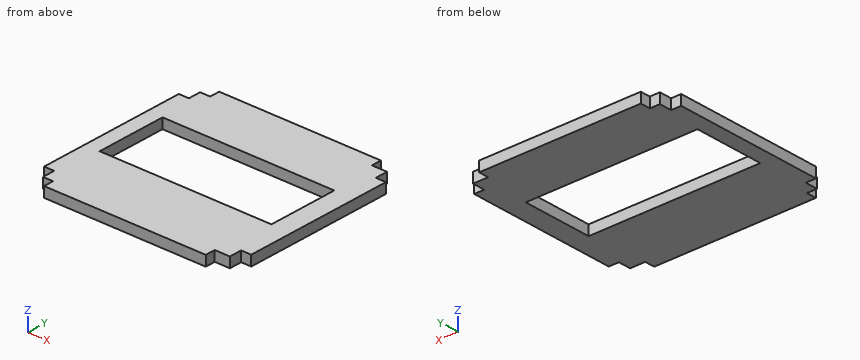
```python
from build123d import *

# Parameters (mm, degrees)
EXTRUDE_1_DEPTH = 2


with BuildPart() as part:
    # 草图1 → 凸台-拉伸1 (new body)
    with BuildSketch(Plane.XY):
        Polygon((0, -35), (2, -35), (2, -37), (34, -37), (34, -35), (37, -35), (37, -32.5), (39, -32.5), (39, -2.5), (37, -2.5), (37, 0), (34, 0), (34, 2), (2, 2), (2, 0), (0, 0), (0, -2.5), (-2, -2.5), (-2, -32.5), (0, -32.5), align=None)
        Polygon((18, -23.5), (2.5, -23.5), (1, -23.5), (1, -11.5), (1, -9.5), (35, -9.5), (35, -11.5), (35, -23.5), (33.5, -23.5), align=None, mode=Mode.SUBTRACT)
    extrude(amount=EXTRUDE_1_DEPTH)


solid = part.part
```
The listing builds one solid part. Answer for the finished solid, in the listing's coordinates (mm). Round coordinates to 2 decimals unless told otherwise and drop trailing zeros. Loops run counter-clockwise (first coordinate to the right, second up) from the corner with the lowest first, then second, coordinate; pieces in that order, holes last.
Q1. Section C-C, the plane y = -15 is taken. Determine the outline of the cut face in (x, z).
Q2. Section A-A, the plane z = 1.4 is taken. Determine the outline of the cut face in (x, y), then the cut area to 3 significant figures.
Q3. Find the intervals of material crossed by line 1 (Y direction, x = 12.5, z = 0.35); line 2 (X direction, y = -23, z = 1.65); line 3 (X direction, y = -0.5, z = 0.5), in increasing order.
Q4. Section B-B, the plane x = 33 is taken. Determine the outline of the cut face in (y, z).
Q5. Section D-D, the plane y = -34 is taken. Determine the outline of the cut face in (x, z).
Q6. Given pin 1 Ø0.6 at (y, z) = (-35.5, 1) entering from -X; pin 2 Ø0.6 at (x, z) = (1, 0.5) entering from -Y; pin 3 Ø1 at (y, z) = (-34.5, 1) entering from +X; pin 4 Ø5 at (x, y) = (14.5, -12.5) entering from +Z, each flat-ended and moving along its own axis, determine where each tip first touches the part or whether it passes through.
Completed:
1. outline: (-2, 0) - (1, 0) - (1, 2) - (-2, 2) - close; (35, 0) - (39, 0) - (39, 2) - (35, 2) - close
2. outline: (-2, -32.5) - (0, -32.5) - (0, -35) - (2, -35) - (2, -37) - (34, -37) - (34, -35) - (37, -35) - (37, -32.5) - (39, -32.5) - (39, -2.5) - (37, -2.5) - (37, 0) - (34, 0) - (34, 2) - (2, 2) - (2, 0) - (0, 0) - (0, -2.5) - (-2, -2.5) - close; hole (1, -23.5) - (35, -23.5) - (35, -9.5) - (1, -9.5) - close
2. area: 1,070 mm2
3. line 1: y = -37 to -23.5, -9.5 to 2
3. line 2: x = -2 to 1, 35 to 39
3. line 3: x = 0 to 37
4. outline: (-37, 0) - (-23.5, 0) - (-23.5, 2) - (-37, 2) - close; (-9.5, 0) - (2, 0) - (2, 2) - (-9.5, 2) - close
5. outline: (0, 0) - (37, 0) - (37, 2) - (0, 2) - close
6. pin 1: stops at x = 2
6. pin 2: stops at y = -35
6. pin 3: stops at x = 37
6. pin 4: passes through
